The drawing under review shows one solid part. Ordinate dimensions are in mm from its lowest x, y, z. Coordinates: 2 decimals unless noted, no trailing zeros. Write each loop counter-clockwise with the first axis right and the second up, starting at its lowest first coordinate (ties: lowest second). Pieces come first, ordered by that corner, then holes.
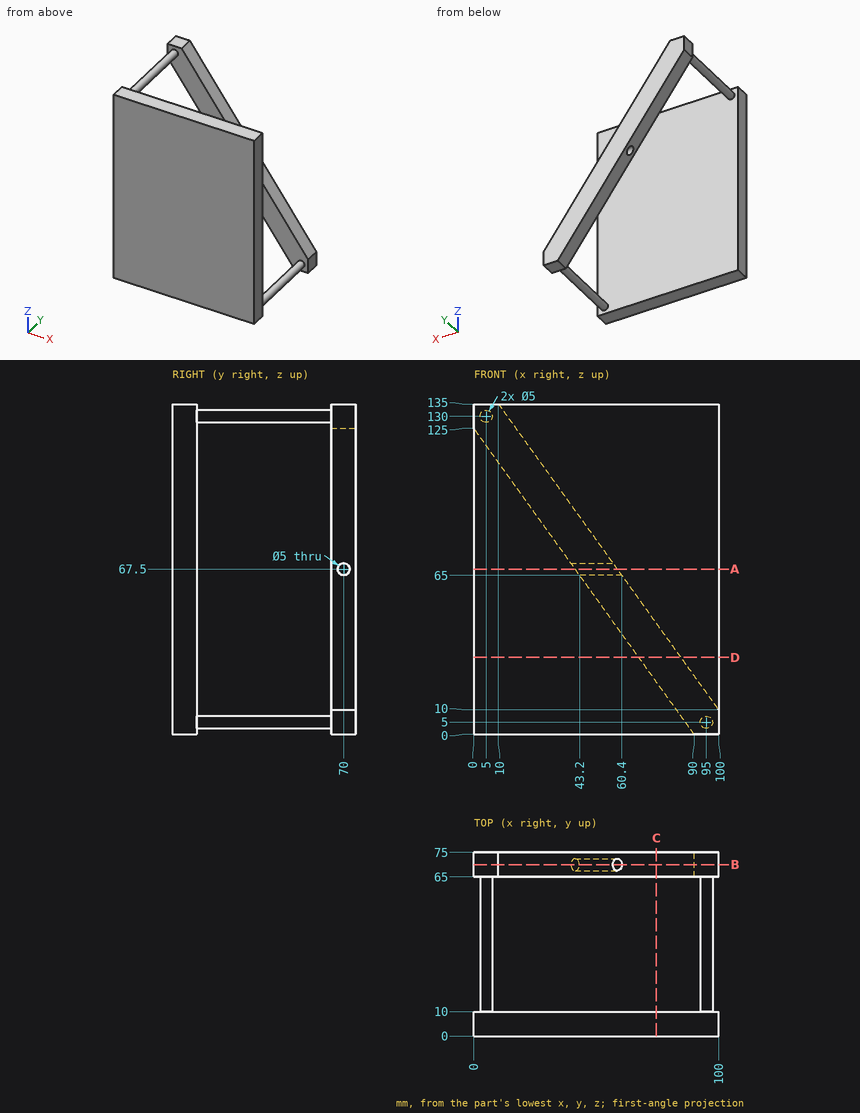
1) Consider section D-D (z = 31.5). Give the boundary of the cut face in (x, y).
2) Clearance check with a flat-ended pin moving along its axis: P1, Ø3, axis at y = 70, z = 67.5, coming from the +X side. State where the tip first meets the part, or that it passes through.
3) Consider section B-B (y = 70). Give the boundary of the cut face in (x, z).
4) Consider section C-C (x = 74.5). Give the boundary of the cut face in (y, z), then the cut area to 3 significant figures.
5) For L1, parallel to Y at x = 47.75, z = 67.5; L2, parallel to Y at x = 49, z = 67; L3, parallel to Y at x = 6.5, z = 12, list the stretches that pass through material, from the lowest coordinate up.
6) Consider section A-A (z = 67.5). Give the boundary of the cut face in (x, y).
Results:
1. outline: (0, 0) - (100, 0) - (100, 10) - (0, 10) - close; (67.32, 65) - (84.52, 65) - (84.52, 75) - (67.32, 75) - close
2. P1: passes through
3. outline: (0, 125) - (39.6, 70) - (56.8, 70) - (10, 135) - (0, 135) - close; (43.2, 65) - (90, 0) - (100, 0) - (100, 10) - (60.4, 65) - close
4. outline: (0, 0) - (10, 0) - (10, 135) - (0, 135) - close; (65, 21.53) - (75, 21.53) - (75, 45.42) - (65, 45.42) - close
4. area: 1,590 mm2
5. L1: y = 0 to 10, 65 to 67.5, 72.5 to 75
5. L2: y = 0 to 10, 65 to 67.55, 72.45 to 75
5. L3: y = 0 to 10
6. outline: (0, 0) - (100, 0) - (100, 10) - (0, 10) - close; (41.4, 65) - (58.6, 65) - (58.6, 67.5) - (41.4, 67.5) - close; (41.4, 72.5) - (58.6, 72.5) - (58.6, 75) - (41.4, 75) - close
